from build123d import *

# Parameters (mm, degrees)
SKETCH1_W           = 200
SKETCH1_H           = 20
BOSS_EXTRUDE1_DEPTH = 3
CUT_EXTRUDE1_REACH  = 102.544
SKETCH2_R           = 1.5
LPATTERN1_COUNT     = 4
LPATTERN1_PITCH     = 64
SKETCH3_W           = 200
SKETCH3_H           = 3
BOSS_EXTRUDE2_DEPTH = 68.54
SKETCH4_W           = 200
SKETCH4_H           = 5
BOSS_EXTRUDE3_DEPTH = 5
SKETCH5_W           = 200
SKETCH5_H           = 12
BOSS_EXTRUDE4_DEPTH = 3
FILLET4_R           = 12
SKETCH6_W           = 3
SKETCH6_H           = 63.54
BOSS_EXTRUDE5_DEPTH = 20
CUT_EXTRUDE2_REACH  = 213.818
SKETCH7_R           = 1.5
CUT_EXTRUDE3_REACH  = 125.397
SKETCH8_R           = 1.5
LPATTERN2_COUNT     = 4
LPATTERN2_PITCH     = 60


with BuildPart() as part:
    # Sketch1 → Boss-Extrude1 (new body)
    with BuildSketch(Plane(origin=(0, 0, 0), x_dir=(1, 0, 0), z_dir=(0, 1, 0))):
        Rectangle(SKETCH1_W, SKETCH1_H)
    extrude(amount=BOSS_EXTRUDE1_DEPTH)

    # Sketch2 → Cut-Extrude1 (cut, up to next)
    with BuildSketch(Plane(origin=(0, 3, 0), x_dir=(1, 0, 0), z_dir=(0, 1, 0)), mode=Mode.PRIVATE) as cut_extrude1_sk1:
        with Locations(Location((-96, 6, 0), (0, 0, 270))):
            Circle(SKETCH2_R)
    cut_extrude1_tool1 = extrude(cut_extrude1_sk1.sketch, amount=-CUT_EXTRUDE1_REACH, mode=Mode.PRIVATE) & part.part
    cut_extrude1 = cut_extrude1_tool1.solids().sort_by_distance((-96, 3, -6))[0]
    add(cut_extrude1, mode=Mode.SUBTRACT)

    # LPattern1: Cut-Extrude1 ×4
    with Locations(*[(i * LPATTERN1_PITCH, 0, 0) for i in range(1, LPATTERN1_COUNT)]):
        add(cut_extrude1, mode=Mode.SUBTRACT)

    # Sketch3 → Boss-Extrude2 (add)
    with BuildSketch(Plane.XZ):
        with Locations((0, 8.5)):
            Rectangle(SKETCH3_W, SKETCH3_H)
    extrude(amount=BOSS_EXTRUDE2_DEPTH)

    # Sketch4 → Boss-Extrude3 (add)
    with BuildSketch(Plane(origin=(0, 0, 7), x_dir=(-1, 0, 0), z_dir=(0, 0, -1))):
        with Locations((0, -2.5)):
            Rectangle(SKETCH4_W, SKETCH4_H)
    extrude(amount=BOSS_EXTRUDE3_DEPTH)

    # Sketch5 → Boss-Extrude4 (add)
    with BuildSketch(Plane(origin=(0, 3, 0), x_dir=(1, 0, 0), z_dir=(0, 1, 0))):
        with Locations((0, -4)):
            Rectangle(SKETCH5_W, SKETCH5_H)
    extrude(amount=BOSS_EXTRUDE4_DEPTH)

    # Fillet4
    fillet4_edges = [part.edges().sort_by_distance(p)[0] for p in [
        (0, 6, 10),
    ]]
    fillet(fillet4_edges, radius=FILLET4_R - 0.0001)  # a hair under: the kernel refuses the full size

    # Sketch6 → Boss-Extrude5 (add)
    with BuildSketch(Plane(origin=(0, 0, 7), x_dir=(-1, 0, 0), z_dir=(0, 0, -1))):
        with Locations((98.5, -36.77)):
            Rectangle(SKETCH6_W, SKETCH6_H)
    extrude(amount=BOSS_EXTRUDE5_DEPTH)

    # Sketch7 → Cut-Extrude2 (cut, up to next)
    with BuildSketch(Plane.ZY.offset(100), mode=Mode.PRIVATE) as cut_extrude2_sk1:
        with Locations((-5, -10.27)):
            Circle(SKETCH7_R)
    cut_extrude2_tool1 = extrude(cut_extrude2_sk1.sketch, amount=-CUT_EXTRUDE2_REACH, mode=Mode.PRIVATE) & part.part
    # Sketch7 → Cut-Extrude2 (cut, up to next)
    with BuildSketch(Plane.ZY.offset(100), mode=Mode.PRIVATE) as cut_extrude2_sk2:
        with Locations((-5, -55.27)):
            Circle(SKETCH7_R)
    cut_extrude2_tool2 = extrude(cut_extrude2_sk2.sketch, amount=-CUT_EXTRUDE2_REACH, mode=Mode.PRIVATE) & part.part
    add(cut_extrude2_tool1.solids().sort_by_distance((-100, -10.27, -5))[0], mode=Mode.SUBTRACT)
    add(cut_extrude2_tool2.solids().sort_by_distance((-100, -55.27, -5))[0], mode=Mode.SUBTRACT)

    # Sketch8 → Cut-Extrude3 (cut, up to next)
    with BuildSketch(Plane.XY.offset(10), mode=Mode.PRIVATE) as cut_extrude3_sk1:
        with Locations((-90, -61.04)):
            Circle(SKETCH8_R)
    cut_extrude3_tool1 = extrude(cut_extrude3_sk1.sketch, amount=-CUT_EXTRUDE3_REACH, mode=Mode.PRIVATE) & part.part
    cut_extrude3 = cut_extrude3_tool1.solids().sort_by_distance((-90, -61.04, 10))[0]
    add(cut_extrude3, mode=Mode.SUBTRACT)

    # LPattern2: Cut-Extrude3 ×4
    with Locations(*[(i * LPATTERN2_PITCH, 0, 0) for i in range(1, LPATTERN2_COUNT)]):
        add(cut_extrude3, mode=Mode.SUBTRACT)


solid = part.part
Source: CAD feature listing. Evaluate the final solid. Frame: model axes, mm. A direction names the side the tool comes from. Give positions to 0.01 mm unless a question says otherwise; leave off trailing zeros. Write each loop counter-clockwise with the first axis right and the second up, starting at its lowest first coordinate (ties: lowest second). Pieces come first, ordered by that corner, then holes. Notation, with made-up numbers: (48, 79) -> (61, 79) arc R16 cw to (61, 101) -> close; hole circle Ø1 at (-1, -14.75). An arc over 180 degrees is marked (long way). Write item = value, one per line.
Q1. First-contact query: pin 1 (5 mm diameter, centred on x = -96, z = -6, fed in from +Y); pin 2 (1.8 mm diameter, centred on x = 30, y = -61.04, fed in from -Z); pin 3 (6 mm diameter, centred on x = -50, y = -12, fed in from -Z); pin 4 (1.5 mm diameter, centred on x = 44.5, z = 5.5, fed in from -Y). Flat tips, straight axial feed; report the tip coordinate or a pass-through.
Here are the results:
pin_1 = 3
pin_2 = through
pin_3 = 7
pin_4 = -5
Q2. Line query: line 1 (X direction, y = 1.2, z = -6); line 2 (Y direction, x = -98.3, z = -5); line 3 (X direction, y = -45, z = -11.5). Output: solid intervals per line, ascending. Write a range as from..to.
Here are the results:
line_1 = -100..-97.5, -94.5..-33.5, -30.5..30.5, 33.5..94.5, 97.5..100
line_2 = -68.54..-56.77, -53.77..-11.77, -8.77..-5, 0..3
line_3 = -100..-97
Q3. Cut plane B-B on y = -26. Return loops of the section in (x, z).
Here are the results:
outline = (-100, -13) -> (-97, -13) -> (-97, 7) -> (100, 7) -> (100, 10) -> (-100, 10) -> close
Q4. Reachability of faces 1 (the face through (-97, -37, -3)), 2 (the face through (-1, 3, -6)), 3 (the face through (1.4, 2.39, 6.58)) from +Z, -Z, +X, -X, +Y, -Y: full face, straight path, thin tool, end or side. Return the list, or none.
Here are the results:
face_1 = -Z, +X, -Y
face_2 = -Z, +X, -X, +Y
face_3 = +Z, +X, -X, +Y
